Geometry: final body of the model. Coordinates: model frame, mm. Face numbers are marked on the shaded views. A direction names the side the tool comes from. Give positions to 0.01 mm unless a question says otherwise; leave off trailing zeros. Write each loop counter-clockwise with the first axis right and the second up, starting at its lowest first coordinate (ties: lowest second). Pieces come first, ordered by that corner, then holes. Notation, with made-up numbers: (75, 70.5) -> (97, 70.5) arc R9 cw to (97, 80.5) -> close; hole circle Ø9 at (-4.75, 17). An arc over 180 degrees is marked (long way). Answer as a JSON object with one key per item and string values.
from build123d import *

# Parameters (mm, degrees)
SKETCH1_W           = 24
SKETCH1_H           = 18
BOSS_EXTRUDE1_DEPTH = 7
FILLET2_R           = 2
SKETCH2_R           = 1.5
SKETCH2_R_2         = 1
BOSS_EXTRUDE2_DEPTH = 4
SKETCH3_R           = 1.5
SKETCH3_R_2         = 1
SKETCH3_W           = 4.5
SKETCH3_H           = 1.5
BOSS_EXTRUDE3_DEPTH = 4


with BuildPart() as part:
    # Sketch1 → Boss-Extrude1 (new body)
    with BuildSketch(Plane(origin=(0, 0, 0), x_dir=(1, 0, 0), z_dir=(0, 1, 0))):
        Rectangle(SKETCH1_W, SKETCH1_H)
    extrude(amount=BOSS_EXTRUDE1_DEPTH)

    # Fillet2
    fillet2_edges = [part.edges().sort_by_distance(p)[0] for p in [
        (-12, 7, 0),
        (0, 7, 9),
        (12, 7, 0),
        (0, 0, 9),
        (-12, 0, 0),
        (0, 0, -9),
        (12, 0, 0),
        (12, 3.5, 9),
        (-12, 3.5, 9),
        (-12, 3.5, -9),
        (12, 3.5, -9),
        (0, 7, -9),
    ]]
    fillet(fillet2_edges, radius=FILLET2_R)

    # Sketch2 → Boss-Extrude2 (add)
    with BuildSketch(Plane(origin=(12, 0, 0), x_dir=(0, 0, -1), z_dir=(1, 0, 0))):
        with Locations((-5.5, 3.5)):
            Circle(SKETCH2_R)
        with Locations((-5.5, 3.5)):
            Circle(SKETCH2_R_2, mode=Mode.SUBTRACT)
        with Locations((0, 3.5)):
            Circle(SKETCH2_R)
        with Locations((0, 3.5)):
            Circle(SKETCH2_R_2, mode=Mode.SUBTRACT)
        with Locations((5.5, 3.5)):
            Circle(SKETCH2_R)
        with Locations((5.5, 3.5)):
            Circle(SKETCH2_R_2, mode=Mode.SUBTRACT)
    extrude(amount=BOSS_EXTRUDE2_DEPTH)

    # Sketch3 → Boss-Extrude3 (add)
    with BuildSketch(Plane.ZY.offset(12)):
        with Locations((-5.5, 3.5)):
            Circle(SKETCH3_R)
        with Locations((-5.5, 3.5)):
            Circle(SKETCH3_R_2, mode=Mode.SUBTRACT)
        with Locations((-1.1, 3.5)):
            Circle(SKETCH3_R)
        with Locations((-1.1, 3.5)):
            Circle(SKETCH3_R_2, mode=Mode.SUBTRACT)
        with Locations((3.75, 3.5)):
            Rectangle(SKETCH3_W, SKETCH3_H)
    extrude(amount=BOSS_EXTRUDE3_DEPTH)


solid = part.part
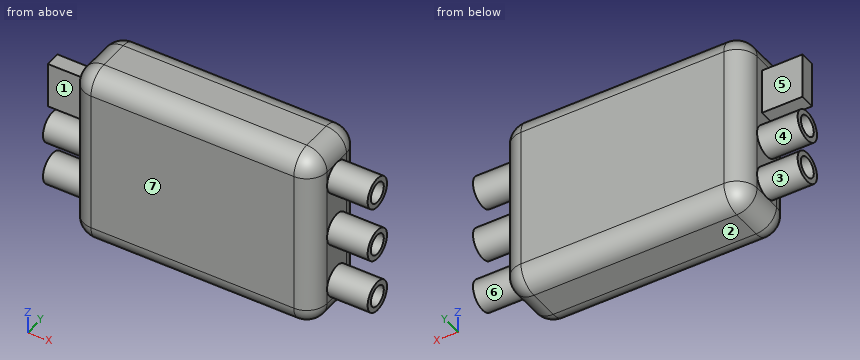
Q1. Cut plane C-C (y = 6.5). Return the cut outline in (x, z), and give its area (3 significant figures).
Values:
{"outline": "(-11.32, -7) arc R1.32 ccw to (-10, -8.32) -> (10, -8.32) arc R1.32 ccw to (11.32, -7) -> (11.32, 7) arc R1.32 ccw to (10, 8.32) -> (-10, 8.32) arc R1.32 ccw to (-11.32, 7) -> close", "area": "375 mm²"}
Q2. Set-up query: the marked faces 4, 5, 6 and 7. Return all of +Z, -Z, +X, -X, +Y, -Y with unobstructed straight access to the full face (end or side cutting, diameter ignored); none if empty.
Values:
{"face 4": "-X", "face 5": "+Z, -X, +Y", "face 6": "+X", "face 7": "+Z, -Z, +X, -X, -Y"}
Q3. First-contact query: P1, Ø1.2, axis at x = -14.5, y = 3, coming from the +Z side; P2, Ø2.5, axis at y = 3.5, z = -2.5, coming from the +X side; P3, Ø1.2, axis at y = 3.5, z = -5.5, coming from the +X side; P4, Ø1.6, axis at x = -13.5, y = 3.5, coming from the -Z side. Flat tips, straight axial feed; report the tip coordinate or a pass-through.
Values:
{"P1": "z = 6", "P2": "x = 16", "P3": "x = 12", "P4": "z = -7"}
Q4. Cut plane A-A (z = 2). Return the cut outline in (x, y).
Values:
{"outline": "(-16, 2.75) -> (-12, 2.75) -> (-12, 2) arc R2 ccw to (-10, 0) -> (10, 0) arc R2 ccw to (12, 2) -> (12, 5) arc R2 ccw to (10, 7) -> (-10, 7) arc R2 ccw to (-12, 5) -> (-12, 4.25) -> (-16, 4.25) -> close"}
Q5. Material intervals for L1, parallel to Y at x = 13.8, z = 5.5; L2, parallel to X at y = 4.25, z = -1.25; L3, parallel to X at y = 2, z = 6.25, sorted ascending. Write a range as from..to.
Values:
{"L1": "2..2.5, 4.5..5", "L2": "-12..16", "L3": "-12..12"}
Q6. Cut plane B-B (x = -6). Return the cut outline in (y, z).
Values:
{"outline": "(0, -7) arc R2 ccw to (2, -9) -> (5, -9) arc R2 ccw to (7, -7) -> (7, 7) arc R2 ccw to (5, 9) -> (2, 9) arc R2 ccw to (0, 7) -> close"}
Q7. Mould query, pull axis Z, two halves, no side actions, for the marked faces 1, 2 and 3. Classes: pulls with the +Z half, pulls with the -Z half, needs draft (parallel to the pull), parting line crosses it, or undercut.
Values:
{"face 1": "needs draft", "face 2": "pulls with the -Z half", "face 3": "undercut"}
